Verification items for the finished model (mm, model axes). Round coordinates to 2 decimals unless told otherwise and drop trailing zeros. Write each loop counter-clockwise with the first axis right and the second up, starting at its lowest first coordinate (ties: lowest second). Pieces come first, ordered by that corner, then holes.
from build123d import *

# Parameters (mm, degrees)
BOSS_EXTRUDE2_DEPTH = 3.175


with BuildPart() as part:
    # Sketch1 → Boss-Extrude2 (new body)
    with BuildSketch(Plane(origin=(0, 0, 0), x_dir=(1, 0, 0), z_dir=(0, 1, 0))):
        with BuildLine():
            Line((0, 0), (127, 0))
            Line((127, 0), (127, 88.516943855))
            ThreePointArc((127, 88.516943855), (126.559592816, 95.191628223), (125.246007425, 101.750581135))
            Line((125.246007425, 101.750581135), (97.832205198, 203.350581135))
            ThreePointArc((97.832205198, 203.350581135), (63.5, 229.647035039), (29.167794802, 203.350581135))
            Line((29.167794802, 203.350581135), (1.753992575, 101.750581135))
            ThreePointArc((1.753992575, 101.750581135), (0.440407184, 95.191628223), (0, 88.516943855))
            Line((0, 88.516943855), (0, 0))
        make_face()
    extrude(amount=BOSS_EXTRUDE2_DEPTH)


solid = part.part
Q1. Sectioned sample at B-B (z = -200). Enter the section's corners in (x, y) (3 decimals).
Recorded:
outline: (28.264, 0) - (98.736, 0) - (98.736, 3.175) - (28.264, 3.175) - close
Q2. Depth check by flat-ended pin: P1, Ø1.5, axis at y = 2, z = -108, coming from the -X side. Enter the tip coordinate at first touch or a pass-through.
Recorded:
P1: stops at x = 3.24
Q3. Sectioned sample at A-A (y = 0.6). Enter the section's corners in (x, z).
Recorded:
outline: (0, -88.52) arc R50.8 ccw to (1.75, -101.75) - (29.17, -203.35) arc R35.56 ccw to (97.83, -203.35) - (125.25, -101.75) arc R50.8 ccw to (127, -88.52) - (127, 0) - (0, 0) - close
Q4. Material ranges on line 1 along Z through (x, y) = (54.5, 1.85); line 2 along Z through (x, y) = (86.5, 1.75); line 3 along X through (y, z) = (1.7, -92.5), recorded low to high.
Recorded:
line 1: z = -228.49 to 0
line 2: z = -221.21 to 0
line 3: x = 0.16 to 126.84
Q5. Sectioned sample at C-C (x = 92.5). Enter the section's corners in (y, z) (3 decimals), plus the area to 3 significant figures.
Recorded:
outline: (0, -214.666) - (3.175, -214.666) - (3.175, 0) - (0, 0) - close
area: 682 mm2
